Geometry: final body of the model. Coordinates: model frame, mm. A direction names the side the tool comes from. Give positions to 0.01 mm unless a question says otherwise; leave off trailing zeros. Write each loop counter-clockwise with the first axis right and the second up, starting at its lowest first coordinate (ties: lowest second). Pieces come first, ordered by that corner, then holes. Notation, with made-up numbers: M 29.25,0 L 67.25,0 A12 cw 67.25,14 Z; hole C 32.5,-6.75 d2. An arc over 180 degrees is marked long. One line per question, with ' | ' between items.
from build123d import *

# Parameters (mm, degrees)
SKETCH_1_W           = 150
SKETCH_1_H           = 160
EXTRUDE_1_DEPTH      = 7
SKETCH_2_W           = 30
SKETCH_2_H           = 70
CUT_EXTRUDE_1_DEPTH  = 10
SKETCH_3_R           = 1.5
CUT_EXTRUDE_2_DEPTH  = 10
SKETCH_4_R           = 1.5
CUT_EXTRUDE_3_DEPTH  = 10
SKETCH_5_R           = 2.5
CUT_EXTRUDE_4_DEPTH  = 3
SKETCH_6_R           = 1.5
CUT_EXTRUDE_5_DEPTH  = 10
CUT_EXTRUDE_6_DEPTH  = 0.5
SKETCH_10_W          = 70
SKETCH_10_H          = 3
EXTRUDE_2_DEPTH      = 10
CUT_EXTRUDE_11_DEPTH = 3
SKETCH_13_W          = 150
SKETCH_13_H          = 7
EXTRUDE_4_DEPTH      = 13
SKETCH_14_W          = 25
SKETCH_14_H          = 5
EXTRUDE_5_DEPTH      = 10
SKETCH_17_W          = 150
SKETCH_17_H          = 7
EXTRUDE_6_DEPTH      = 8
SKETCH_19_W          = 7
SKETCH_19_H          = 76
EXTRUDE_8_DEPTH      = 8
SKETCH_20_W          = 7
SKETCH_20_H          = 76
EXTRUDE_9_DEPTH      = 8
CUT_EXTRUDE_14_DEPTH = 3
SKETCH_27_W          = 7
SKETCH_27_H          = 35
EXTRUDE_14_DEPTH     = 8
SKETCH_28_W          = 7
SKETCH_28_H          = 35
EXTRUDE_15_DEPTH     = 8
CUT_EXTRUDE_15_DEPTH = 3
CUT_EXTRUDE_16_DEPTH = 2
SKETCH_30_R          = 1.6
CUT_EXTRUDE_17_DEPTH = 7
SKETCH_31_R          = 3.1
CUT_EXTRUDE_18_DEPTH = 3.5
SKETCH_32_R          = 2.5
CUT_EXTRUDE_19_DEPTH = 4


with BuildPart() as part:
    # 草圖1 → 填料-伸長1 (new body)
    with BuildSketch(Plane.XY):
        Rectangle(SKETCH_1_W, SKETCH_1_H)
    extrude(amount=EXTRUDE_1_DEPTH)

    # 草圖2 → 除料-伸長1 (cut)
    with BuildSketch(Plane(origin=(0, 0, 0), x_dir=(-1, 0, 0), z_dir=(0, 0, -1))):
        with Locations((-60, -23)):
            Rectangle(SKETCH_2_W, SKETCH_2_H)
        with Locations((60, -23)):
            Rectangle(SKETCH_2_W, SKETCH_2_H)
    extrude(amount=-CUT_EXTRUDE_1_DEPTH, mode=Mode.SUBTRACT)

    # 草圖3 → 除料-伸長2 (cut)
    with BuildSketch(Plane(origin=(0, 0, 0), x_dir=(-1, 0, 0), z_dir=(0, 0, -1))):
        with Locations((-35, -25.75)):
            Circle(SKETCH_3_R)
        with Locations((-23, -25.75)):
            Circle(SKETCH_3_R)
        with Locations((-35.024958581, -49.749987022)):
            Circle(SKETCH_3_R)
        with Locations((-23.024958581, -49.749987022)):
            Circle(SKETCH_3_R)
    extrude(amount=-CUT_EXTRUDE_2_DEPTH, mode=Mode.SUBTRACT)

    # 草圖4 → 除料-伸長3 (cut)
    with BuildSketch(Plane(origin=(0, 0, 0), x_dir=(-1, 0, 0), z_dir=(0, 0, -1))):
        with Locations((35, -25.75)):
            Circle(SKETCH_4_R)
        with Locations((23, -25.75)):
            Circle(SKETCH_4_R)
        with Locations((35, -49.75)):
            Circle(SKETCH_4_R)
        with Locations((23, -49.75)):
            Circle(SKETCH_4_R)
    extrude(amount=-CUT_EXTRUDE_3_DEPTH, mode=Mode.SUBTRACT)

    # 草圖5 → 除料-伸長4 (cut)
    with BuildSketch(Plane.XY.offset(7)):
        with Locations((-35, -25.75)):
            Circle(SKETCH_5_R)
        with Locations((-23, -25.75)):
            Circle(SKETCH_5_R)
        with Locations((-35, -49.75)):
            Circle(SKETCH_5_R)
        with Locations((-23, -49.75)):
            Circle(SKETCH_5_R)
        with Locations((23.024958581, -49.749987022)):
            Circle(SKETCH_5_R)
        with Locations((35.024958581, -49.749987022)):
            Circle(SKETCH_5_R)
        with Locations((35, -25.75)):
            Circle(SKETCH_5_R)
        with Locations((23, -25.75)):
            Circle(SKETCH_5_R)
    extrude(amount=-CUT_EXTRUDE_4_DEPTH, mode=Mode.SUBTRACT)

    # 草圖6 → 除料-伸長5 (cut)
    with BuildSketch(Plane(origin=(0, 0, 0), x_dir=(-1, 0, 0), z_dir=(0, 0, -1))):
        with Locations((-14.13500283, 66.177513248)):
            Circle(SKETCH_6_R)
        with Locations((9.86499717, 66.177513248)):
            Circle(SKETCH_6_R)
        with Locations((9.86499717, 54.177513248)):
            Circle(SKETCH_6_R)
        with Locations((-14.13500283, 54.177513248)):
            Circle(SKETCH_6_R)
    extrude(amount=-CUT_EXTRUDE_5_DEPTH, mode=Mode.SUBTRACT)

    # 草圖7 → 除料-伸長6 (cut)
    with BuildSketch(Plane(origin=(0, 0, 0), x_dir=(-1, 0, 0), z_dir=(0, 0, -1))):
        Polygon((72.33, -65), (70.54, -61.899629054), (66.96, -61.899629054), (65.17, -65), (66.96, -68.100370946), (70.54, -68.100370946), align=None)
        Polygon((72.33, 65), (70.54, 68.100370946), (66.96, 68.100370946), (65.17, 65), (66.96, 61.899629054), (70.54, 61.899629054), align=None)
        Polygon((-65.17, 65), (-66.96, 68.100370946), (-70.54, 68.100370946), (-72.33, 65), (-70.54, 61.899629054), (-66.96, 61.899629054), align=None)
        Polygon((-65.17, -65), (-66.96, -61.899629054), (-70.54, -61.899629054), (-72.33, -65), (-70.54, -68.100370946), (-66.96, -68.100370946), align=None)
    extrude(amount=-CUT_EXTRUDE_6_DEPTH, mode=Mode.SUBTRACT)

    # 草圖10 → 填料-伸長2 (add)
    with BuildSketch(Plane(origin=(0, 0, 0), x_dir=(-1, 0, 0), z_dir=(0, 0, -1))):
        with Locations((0, 71.189628596)):
            Rectangle(SKETCH_10_W, SKETCH_10_H)
    extrude(amount=EXTRUDE_2_DEPTH)

    # 草圖11 → 除料-伸長11 (cut)
    with BuildSketch(Plane(origin=(0, 0, 0), x_dir=(-1, 0, 0), z_dir=(0, 0, -1))):
        with BuildLine():
            Line((-35, 12), (35, 12))
            ThreePointArc((35, 12), (42.071067812, 9.071067812), (45, 2))
            Line((45, 2), (45, -58))
            Line((45, -58), (-45, -58))
            Line((-45, -58), (-45, 2))
            ThreePointArc((-45, 2), (-42.071067812, 9.071067812), (-35, 12))
        make_face()
    extrude(amount=-CUT_EXTRUDE_11_DEPTH, mode=Mode.SUBTRACT)

    # 草圖13 → 填料-伸長4 (add)
    with BuildSketch(Plane.XZ.offset(80)):
        with Locations((0, 3.5)):
            Rectangle(SKETCH_13_W, SKETCH_13_H)
    extrude(amount=EXTRUDE_4_DEPTH)

    # 草圖14 → 填料-伸長5 (add)
    with BuildSketch(Plane(origin=(0, 0, 0), x_dir=(-1, 0, 0), z_dir=(0, 0, -1))):
        with Locations((-47.5, 14.5)):
            Rectangle(SKETCH_14_W, SKETCH_14_H)
        with Locations((47.5, 14.5)):
            Rectangle(SKETCH_14_W, SKETCH_14_H)
    extrude(amount=EXTRUDE_5_DEPTH)

    # 草圖17 → 填料-伸長6 (add)
    with BuildSketch(Plane(origin=(0, 80, 0), x_dir=(1, 0, 0), z_dir=(0, 1, 0))):
        with Locations((0, -3.5)):
            Rectangle(SKETCH_17_W, SKETCH_17_H)
    extrude(amount=EXTRUDE_6_DEPTH)

    # 草圖19 → 填料-伸長8 (add)
    with BuildSketch(Plane(origin=(75, 0, 0), x_dir=(0, 0, -1), z_dir=(1, 0, 0))):
        with Locations((-3.5, 50)):
            Rectangle(SKETCH_19_W, SKETCH_19_H)
    extrude(amount=EXTRUDE_8_DEPTH)

    # 草圖20 → 填料-伸長9 (add)
    with BuildSketch(Plane.ZY.offset(75)):
        with Locations((3.5, 50)):
            Rectangle(SKETCH_20_W, SKETCH_20_H)
    extrude(amount=EXTRUDE_9_DEPTH)

    # 草圖26 → 除料-伸長14 (cut)
    with BuildSketch(Plane(origin=(0, 0, 0), x_dir=(-1, 0, 0), z_dir=(0, 0, -1))):
        Polygon((-83, 85), (-83, 12), (-74.5, 12), (-74.5, 79.5), (74.5, 79.5), (74.5, 12), (83, 12), (83, 85), align=None)
    extrude(amount=-CUT_EXTRUDE_14_DEPTH, mode=Mode.SUBTRACT)

    # 草圖27 → 填料-伸長14 (add)
    with BuildSketch(Plane(origin=(75, 0, 0), x_dir=(0, 0, -1), z_dir=(1, 0, 0))):
        with Locations((-3.5, -75.5)):
            Rectangle(SKETCH_27_W, SKETCH_27_H)
    extrude(amount=EXTRUDE_14_DEPTH)

    # 草圖28 → 填料-伸長15 (add)
    with BuildSketch(Plane.ZY.offset(75)):
        with Locations((3.5, -75.5)):
            Rectangle(SKETCH_28_W, SKETCH_28_H)
    extrude(amount=EXTRUDE_15_DEPTH)

    # 草圖29 → 除料-伸長15 (cut)
    with BuildSketch(Plane(origin=(0, 0, 0), x_dir=(-1, 0, 0), z_dir=(0, 0, -1))):
        Polygon((83, -58), (83, -90), (-83, -90), (-83, -58), (-74.841372547, -58), (-74.841372547, -84.5), (74.158627453, -84.5), (74.158627453, -58), align=None)
    extrude(amount=-CUT_EXTRUDE_15_DEPTH, mode=Mode.SUBTRACT)

    # 草圖8 → 除料-伸長16 (cut)
    with BuildSketch(Plane(origin=(0, 0, 0.5), x_dir=(-1, 0, 0), z_dir=(0, 0, -1))):
        Polygon((-65.75, 65), (-67.25, 67.598076211), (-70.25, 67.598076211), (-71.75, 65), (-70.25, 62.401923789), (-67.25, 62.401923789), align=None)
        Polygon((71.75, 65), (70.25, 67.598076211), (67.25, 67.598076211), (65.75, 65), (67.25, 62.401923789), (70.25, 62.401923789), align=None)
        Polygon((-65.75, -65), (-67.25, -62.401923789), (-70.25, -62.401923789), (-71.75, -65), (-70.25, -67.598076211), (-67.25, -67.598076211), align=None)
        Polygon((71.75, -65), (70.25, -62.401923789), (67.25, -62.401923789), (65.75, -65), (67.25, -67.598076211), (70.25, -67.598076211), align=None)
    extrude(amount=-CUT_EXTRUDE_16_DEPTH, mode=Mode.SUBTRACT)

    # 草圖30 → 除料-伸長17 (cut)
    with BuildSketch(Plane.XY):
        with Locations(Location((68.75, -65, 0), (0, 0, 180))):
            Circle(SKETCH_30_R)
        with Locations(Location((68.75, 65, 0), (0, 0, 180))):
            Circle(SKETCH_30_R)
        with Locations(Location((-68.75, -65, 0), (0, 0, 180))):
            Circle(SKETCH_30_R)
        with Locations(Location((-68.75, 65, 0), (0, 0, 180))):
            Circle(SKETCH_30_R)
    extrude(amount=CUT_EXTRUDE_17_DEPTH, mode=Mode.SUBTRACT)

    # 草圖31 → 除料-伸長18 (cut)
    with BuildSketch(Plane.XY.offset(7)):
        with Locations((-68.75, 65)):
            Circle(SKETCH_31_R)
        with Locations((-68.75, -65)):
            Circle(SKETCH_31_R)
        with Locations((68.75, -65)):
            Circle(SKETCH_31_R)
        with Locations((68.75, 65)):
            Circle(SKETCH_31_R)
    extrude(amount=-CUT_EXTRUDE_18_DEPTH, mode=Mode.SUBTRACT)

    # 草圖32 → 除料-伸長19 (cut)
    with BuildSketch(Plane(origin=(0, 0, 0), x_dir=(-1, 0, 0), z_dir=(0, 0, -1))):
        with Locations((-14.13500283, 66.177513248)):
            Circle(SKETCH_32_R)
        with Locations((-14.13500283, 54.177513248)):
            Circle(SKETCH_32_R)
        with Locations((9.86499717, 54.177513248)):
            Circle(SKETCH_32_R)
        with Locations((9.86499717, 66.177513248)):
            Circle(SKETCH_32_R)
    extrude(amount=-CUT_EXTRUDE_19_DEPTH, mode=Mode.SUBTRACT)


solid = part.part
(1) Material intervals for L1, parallel to Y at x = -23, z = 3.75; L2, parallel to Y at x = -36.5, z = -8.75; L3, parallel to X at y = 25.5, z = 1, sorted ascending. Write a range as [from, to].
Working result:
L1: y = [-93, -51.25], [-48.25, -27.25], [-24.25, 88] | L2: y = [12, 17] | L3: x = [-74.5, 74.5]
(2) Set-up query: faces 1 (the face through (70.42, -62.39, 5.27)), 2 (the face through (43, 10, 0)), 3 (the face through (53, 12, -1)), 4 (the face through (-35, 14, -5)), 5 (the face through (66, -66, 0.5)). Return all of +Z, -Z, +X, -X, +Y, -Y with unobstructed straight access to the full face (end or side cutting, diameter ignored); none if empty.
Working result:
face 1: +Z | face 2: -Z, +X, -X, -Y | face 3: -Z, +X | face 4: -Z, -Y | face 5: -Z
(3) First-contact query: P1, Ø1.8, axis at x = -35, y = -25.75, coming from the -Z side; P2, Ø7, axis at x = 68.75, y = -65, coming from the -Z side; P3, Ø5, axis at y = -15, z = 3.5, coming from the -X side; P4, Ø4, axis at x = -35, y = -49.75, coming from the -Z side. Flat tips, straight axial feed; report the tip coordinate or a pass-through.
Working result:
P1: passes through | P2: stops at z = 0 | P3: stops at x = -45 | P4: stops at z = 3
(4) Cut plane C-C, the plane x = 30.5. Return loops of the section in (y, z), then the cut area to 3 significant figures.
Working result:
outline: M -93,0 L -90,0 L -90,3 L -84.5,3 L -84.5,0 L -58,0 L -58,3 L 12,3 L 12,0 L 69.69,0 L 69.69,-10 L 72.69,-10 L 72.69,0 L 79.5,0 L 79.5,3 L 85,3 L 85,0 L 88,0 L 88,7 L -93,7 Z | area: 1,050 mm^2
(5) Cut plane A-A, the plane z = -2.5. Return loops of the section in (x, y), then the cut area to 3 significant figures.
Working result:
outline: M -60,12 L -35,12 L -35,17 L -60,17 Z; M -35,69.69 L 35,69.69 L 35,72.69 L -35,72.69 Z; M 35,12 L 60,12 L 60,17 L 35,17 Z | area: 460 mm^2
(6) Cut plane B-B, the plane y = 27. Return loops of the section in (x, z).
Working result:
outline: M -83,3 L -74.5,3 L -74.5,0 L 74.5,0 L 74.5,3 L 83,3 L 83,7 L -83,7 Z
(7) Draft query along X for faces 6 (the face through (-71, -63, 0.5)), 7 (the face through (-47, 17, -5)). Return one class per face: released by +X, released by -X, zero draft, split by the parting line, or undercut.
Working result:
face 6: undercut | face 7: zero draft
